from build123d import *

# Parameters (mm, degrees)
BASE_FLANGE1_DEPTH = 1
CUT_EXTRUDE1_DEPTH = 10
CUT_EXTRUDE2_DEPTH = 10


# Sheet-metal steps are written as plain solids
with BuildPart() as part:
    # Sketch1 → Base-Flange1 (new body)
    with BuildSketch(Plane.XY):
        with BuildLine():
            Line((0, 0), (663.4, 0))
            Line((663.4, 0), (663.4, 992))
            ThreePointArc((663.4, 992), (658.801576465, 1003.101576465), (647.7, 1007.7))
            Line((647.7, 1007.7), (15.7, 1007.7))
            ThreePointArc((15.7, 1007.7), (4.598423535, 1003.101576465), (0, 992))
            Line((0, 992), (0, 0))
        make_face()
    extrude(amount=-BASE_FLANGE1_DEPTH)

    # Sketch9 → Cut-Extrude1 (cut)
    with BuildSketch(Plane.XY):
        with BuildLine():
            Line((562.2, 900.7), (301.2, 900.7))
            ThreePointArc((301.2, 900.7), (299.785786438, 900.114213562), (299.2, 898.7))
            Line((299.2, 898.7), (299.2, 814.7))
            ThreePointArc((299.2, 814.7), (299.785786438, 813.285786438), (301.2, 812.7))
            Line((301.2, 812.7), (562.2, 812.7))
            ThreePointArc((562.2, 812.7), (563.614213562, 813.285786438), (564.2, 814.7))
            Line((564.2, 814.7), (564.2, 898.7))
            ThreePointArc((564.2, 898.7), (563.614213562, 900.114213562), (562.2, 900.7))
        make_face()
        with BuildLine():
            Line((564.2, 718.7), (564.2, 634.7))
            ThreePointArc((564.2, 634.7), (563.614213562, 633.285786438), (562.2, 632.7))
            Line((562.2, 632.7), (301.2, 632.7))
            ThreePointArc((301.2, 632.7), (299.785786438, 633.285786438), (299.2, 634.7))
            Line((299.2, 634.7), (299.2, 718.7))
            ThreePointArc((299.2, 718.7), (299.785786438, 720.114213562), (301.2, 720.7))
            Line((301.2, 720.7), (562.2, 720.7))
            ThreePointArc((562.2, 720.7), (563.614213562, 720.114213562), (564.2, 718.7))
        make_face()
        with BuildLine():
            Line((564.2, 538.7), (564.2, 454.7))
            ThreePointArc((564.2, 454.7), (563.614213562, 453.285786438), (562.2, 452.7))
            Line((562.2, 452.7), (301.2, 452.7))
            ThreePointArc((301.2, 452.7), (299.785786438, 453.285786438), (299.2, 454.7))
            Line((299.2, 454.7), (299.2, 538.7))
            ThreePointArc((299.2, 538.7), (299.785786438, 540.114213562), (301.2, 540.7))
            Line((301.2, 540.7), (562.2, 540.7))
            ThreePointArc((562.2, 540.7), (563.614213562, 540.114213562), (564.2, 538.7))
        make_face()
        with BuildLine():
            Line((564.2, 358.7), (564.2, 274.7))
            ThreePointArc((564.2, 274.7), (563.614213562, 273.285786438), (562.2, 272.7))
            Line((562.2, 272.7), (301.2, 272.7))
            ThreePointArc((301.2, 272.7), (299.785786438, 273.285786438), (299.2, 274.7))
            Line((299.2, 274.7), (299.2, 358.7))
            ThreePointArc((299.2, 358.7), (299.785786438, 360.114213562), (301.2, 360.7))
            Line((301.2, 360.7), (562.2, 360.7))
            ThreePointArc((562.2, 360.7), (563.614213562, 360.114213562), (564.2, 358.7))
        make_face()
        with BuildLine():
            Line((564.2, 178.7), (564.2, 94.7))
            ThreePointArc((564.2, 94.7), (563.614213562, 93.285786438), (562.2, 92.7))
            Line((562.2, 92.7), (301.2, 92.7))
            ThreePointArc((301.2, 92.7), (299.785786438, 93.285786438), (299.2, 94.7))
            Line((299.2, 94.7), (299.2, 178.7))
            ThreePointArc((299.2, 178.7), (299.785786438, 180.114213562), (301.2, 180.7))
            Line((301.2, 180.7), (562.2, 180.7))
            ThreePointArc((562.2, 180.7), (563.614213562, 180.114213562), (564.2, 178.7))
        make_face()
    extrude(amount=-CUT_EXTRUDE1_DEPTH, mode=Mode.SUBTRACT)

    # Sketch10 → Cut-Extrude2 (cut)
    with BuildSketch(Plane.XY):
        with BuildLine():
            Line((65.7, 629.2), (197.7, 629.2))
            ThreePointArc((197.7, 629.2), (204.771067812, 632.128932188), (207.7, 639.2))
            Line((207.7, 639.2), (207.7, 889.2))
            ThreePointArc((207.7, 889.2), (204.771067812, 896.271067812), (197.7, 899.2))
            Line((197.7, 899.2), (65.7, 899.2))
            ThreePointArc((65.7, 899.2), (58.628932188, 896.271067812), (55.7, 889.2))
            Line((55.7, 889.2), (55.7, 639.2))
            ThreePointArc((55.7, 639.2), (58.628932188, 632.128932188), (65.7, 629.2))
        make_face()
    extrude(amount=-CUT_EXTRUDE2_DEPTH, mode=Mode.SUBTRACT)


solid = part.part
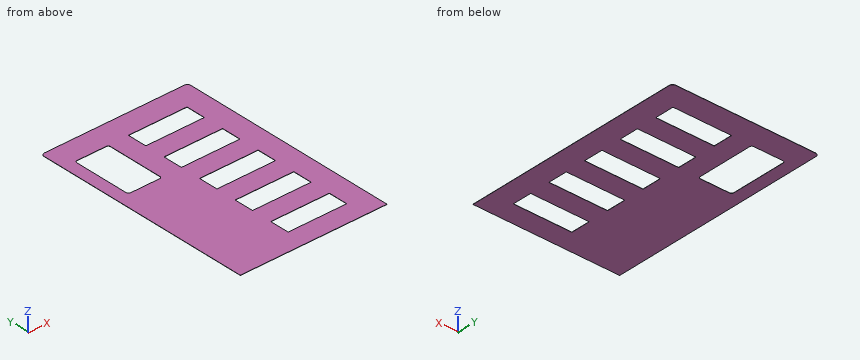
For this review, take the finished solid that the model builds, in its own axes (mm). Give positions to 0.01 mm unless a question says otherwise; leave off trailing zeros. Loops run counter-clockwise (first coordinate to the right, second up) from the corner with the lowest first, then second, coordinate; pieces in that order, holes last. Notation, with made-up numbers: M -39.5,63 L -18.5,63 A21 cw -18.5,91 Z; hole C 74.25,63 d4. An arc over 180 degrees is marked long. Answer as a JSON object with one key per item and string values. Group by question number.
Q1. Add section C-C on z = -0.5. Give the number of separate pieces and of enclosed holes in the cut face, and give its area (3 significant figures).
Q2. Add section A-A on x = 324.5. Give the boundary of the cut face in (y, z).
Q3. Add section B-B on y = 797.5. Give the boundary of the cut face in (x, z), and give its area (3 significant figures).
Q4. For probe 1 along Y at (x, z) = (331.5, -0.35); probe 2 along X at (y, z) = (714, -0.3); probe 3 along Y at (x, z) = (177, -0.35), list the stretches that pass through material, from the lowest coordinate up. Write a range as [from, to].
Checked values:
{
 "1": {"separate pieces": "1", "enclosed holes": "6", "area": "511,000 mm²"},
 "2": {"outline": "M 0,-1 L 92.7,-1 L 92.7,0 L 0,0 Z; M 180.7,-1 L 272.7,-1 L 272.7,0 L 180.7,0 Z; M 360.7,-1 L 452.7,-1 L 452.7,0 L 360.7,0 Z; M 540.7,-1 L 632.7,-1 L 632.7,0 L 540.7,0 Z; M 720.7,-1 L 812.7,-1 L 812.7,0 L 720.7,0 Z; M 900.7,-1 L 1007.7,-1 L 1007.7,0 L 900.7,0 Z"},
 "3": {"outline": "M 0,-1 L 55.7,-1 L 55.7,0 L 0,0 Z; M 207.7,-1 L 663.4,-1 L 663.4,0 L 207.7,0 Z", "area": "511 mm²"},
 "4": {"probe 1": "[0, 92.7], [180.7, 272.7], [360.7, 452.7], [540.7, 632.7], [720.7, 812.7], [900.7, 1007.7]", "probe 2": "[0, 55.7], [207.7, 299.2], [564.2, 663.4]", "probe 3": "[0, 629.2], [899.2, 1007.7]"}
}
